Verification items for this drawing (mm, ordinates from the low corner). A direction names the side the tool comes from. Coordinates: 2 decimals unless noted, no trailing zeros. Write each loop counter-clockwise with the first axis right and the second up, starting at its lowest first coordinate (ties: lowest second). Pieces come first, ordered by that corner, then holes. Notation, with made-up numbers: M 57.25,-2 L 91.25,-2 A26 cw 91.25,14 Z; hole C 14,-0.75 d10. An arc over 180 degrees is marked long. Put each result on its own line as item: value. Start each with the question number.
1) Scan lines: line 1 along Y through (x, z) = (41.65, 42.9); line 2 along X through (y, z) = (5.65, 40.2); line 3 along Y through (x, z) = (10.65, 40.3). Record each from-to range of solid material in increasing order.
2) Cross-section at A-A on x = 26.15. Record the cut outline in (y, z), plus the area to 4 significant figures.
3) Cross-section at B-B on y = 36.65. Record the cut outline in (x, z).
4) Mould release check, pull along Y, two halves, no side actions. Record for the marked faces 1, 2 and 3: released by +Y, released by -Y, zero draft, split by the parting line, or undercut.
5) Cross-section at D-D on y = 21.15. Record the cut outline in (x, z).
6) Cross-section at C-C on x = 41.65. Record the cut outline in (y, z), plus the area to 3 significant figures.
7) Gauge pin test, flat ends, axial feed: pin 1 (5 mm diameter, centred on x = 41.65, y = 36.65, fed in from -Z); pin 2 (8 mm diameter, centred on y = 10.5, z = 23.5, fed in from -X); pin 3 (3 mm diameter, centred on x = 11, y = 4.5, fed in from +Z). Record the tip position at first contact, or that the pin passes through.
8) Set-up check for the marked faces 4 and 5: record each of +Z, -Z, +X, -X, +Y, -Y from which the full face is reachable in a straight line by a thin tool's end or side.
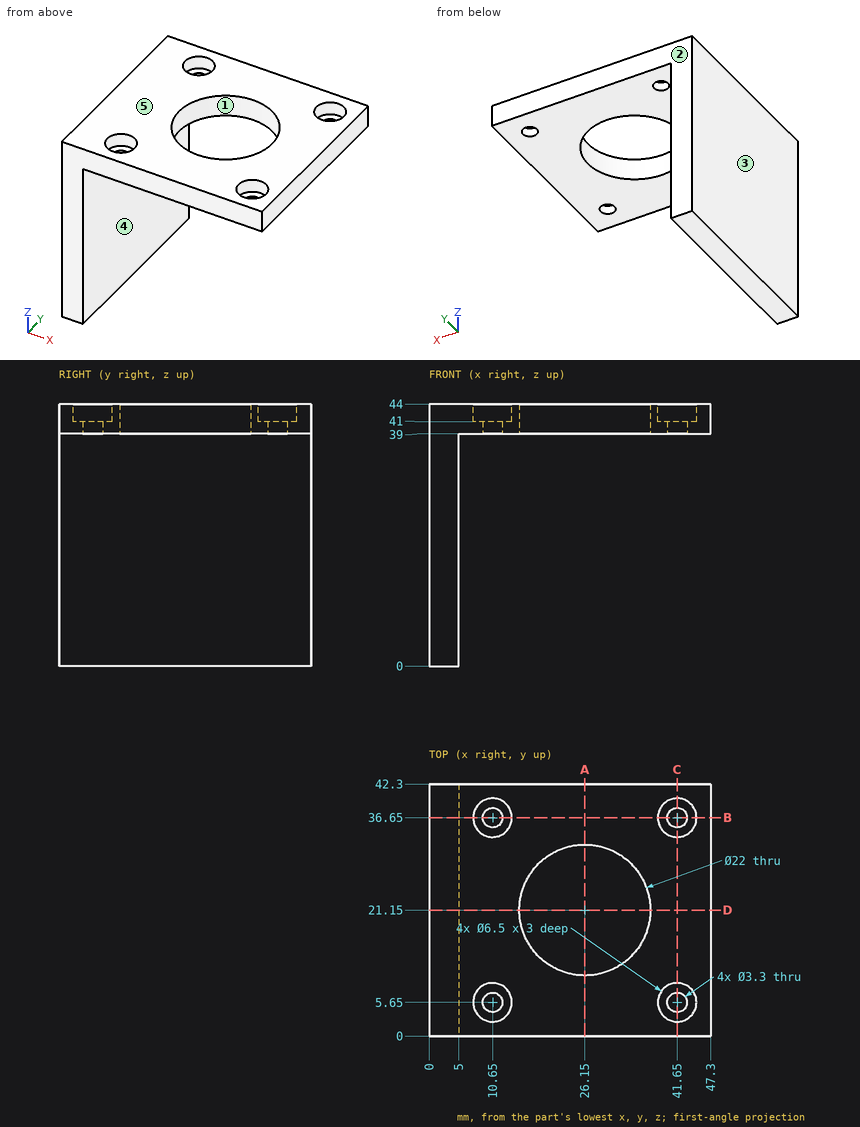
Answer key:
1. line 1: y = 0 to 2.4, 8.9 to 33.4, 39.9 to 42.3
1. line 2: x = 0 to 9, 12.3 to 40, 43.3 to 47.3
1. line 3: y = 0 to 4, 7.3 to 35, 38.3 to 42.3
2. outline: M 0,39 L 10.15,39 L 10.15,44 L 0,44 Z; M 32.15,39 L 42.3,39 L 42.3,44 L 32.15,44 Z
2. area: 101.5 mm²
3. outline: M 0,0 L 5,0 L 5,39 L 9,39 L 9,41 L 7.4,41 L 7.4,44 L 0,44 Z; M 12.3,39 L 40,39 L 40,41 L 38.4,41 L 38.4,44 L 13.9,44 L 13.9,41 L 12.3,41 Z; M 43.3,39 L 47.3,39 L 47.3,44 L 44.9,44 L 44.9,41 L 43.3,41 Z
4. face 1: undercut
4. face 2: released by +Y
4. face 3: zero draft
5. outline: M 0,0 L 5,0 L 5,39 L 15.15,39 L 15.15,44 L 0,44 Z; M 37.15,39 L 47.3,39 L 47.3,44 L 37.15,44 Z
6. outline: M 0,39 L 4,39 L 4,41 L 2.4,41 L 2.4,44 L 0,44 Z; M 7.3,39 L 35,39 L 35,41 L 33.4,41 L 33.4,44 L 8.9,44 L 8.9,41 L 7.3,41 Z; M 38.3,39 L 42.3,39 L 42.3,44 L 39.9,44 L 39.9,41 L 38.3,41 Z
6. area: 159 mm²
7. pin 1: stops at z = 39
7. pin 2: stops at x = 0
7. pin 3: stops at z = 41
8. face 4: -Z, +X, +Y, -Y
8. face 5: +Z, +X, -X, +Y, -Y
